Solid Edge part; units mm, degrees
sketch "Sketch1" plane through (0, 0, 0) normal (0, -1, 0) x (1, 0, 0)
  line L0 (-6.3509, -11) -> (6.3509, -11)
  line L1 (6.3509, -11) -> (12.7017, 0)
  line L2 (12.7017, 0) -> (6.3509, 11)
  line L3 (6.3509, 11) -> (-6.3509, 11)
  line L4 (-6.3509, 11) -> (-12.7017, 0)
  line L5 (-12.7017, 0) -> (-6.3509, -11)
extrude "Protrusion1" add sketch "Sketch1" along normal mid plane 16
sketch "Sketch2" plane through (0, 0, 0) normal (1, 0, 0) x (0, 1, 0)
  line L0 (8, -10) -> (7.2508, -12.391)
revolve "RevolvedCutout1" cut sketch "Sketch2" angle 360 about axis through (0, -63.5, 0) along (0, 1, 0) material side at (0, 7.6731, -11.2105)
mirror "Mirror1" about plane through (0, 0, 0) normal (0, -1, 0) of "RevolvedCutout1"
sketch "Sketch3" plane through (0, 0, 0) normal (1, 0, 0) x (0, 1, 0)
  line L0 (-8, -7.5) -> (-1.9048, -7.5)
  line L1 (-1.9048, -7.5) -> (-1.9048, -6)
  line L2 (-1.9048, -6) -> (7.1535, -6)
revolve "RevolvedCutout3" cut sketch "Sketch3" angle 360 about axis through (0, 7.1535, 0) along (0, -1, 0) material side at (0, -4.9524, -7.45)
Verification items for the finished model (mm, model axes). A direction names the side the tool comes from. Give positions to 0.01 mm unless a question says otherwise; leave off trailing zeros. Order: outer loops, then holes, each group sorted by start corner. A loop starts at its lowest first (then second) coordinate and runs counter-clockwise, first axis right, second up. Notation, with made-up numbers: M -21.75,65 L 22.25,65 A31 ccw 22.25,90 Z; hole C -18,0.5 d10. An arc over 180 degrees is marked long. Answer in a Markdown table with one row per item. Add a question column.
Item 1: Gauge pin test, flat ends, axial feed: pin 1 (7.5 mm diameter, centred on x = 3, z = 1, fed in from -Y); pin 2 (8 mm diameter, centred on x = 9, z = -7, fed in from -Y); pin 3 (4 mm diameter, centred on x = 8.5, y = -3, fed in from -Z). Record the tip position at first contact, or that the pin passes through.
Item 2: Scan lines: probe 1 along Z at (x, y) = (0, 5.25); probe 2 along Z at (x, y) = (-1.5, 5.5); probe 3 along X at (y, z) = (0.5, -1.75). Record each from-to range of solid material in increasing order. Write a range as from..to.
Item 3: Mould release check, pull along X, two halves, no side actions. Record for faces 3 (the flat face through (-9.571, 0.108, -5.423)), 4 (the cylindrical face through (-0.33, -4.91, 7.493)), 5 (the flat face through (0, 0, 11)): released by +X, released by -X, zero draft, split by the parting line, or undercut.
Item 4: Section check A-A, the plane x = 0. Enter the section's corners in (y, z).
Item 5: Section check B-B, the plane y = 3.25. Enter the section's corners in (x, z), and give its area (3 significant figures).
Item 6: Tool access check on faces 1 (the cylindrical face through (0, 3, 6)), 2 (the flat face through (6, -1.905, -2)). Record the directions out of +Z, -Z, +X, -X, +Y, -Y that give a thin tool (end or side, any length) a straight path to the whole face; none if there is none.
Filled sheet:
| question | item | result |
|---|---|---|
| 1 | pin 1 | stops at y = -1.9 |
| 1 | pin 2 | stops at y = -8 |
| 1 | pin 3 | stops at z = -10.74 |
| 2 | probe 1 | z = -11..-6, 6..11 |
| 2 | probe 2 | z = -11..-5.81, 5.81..11 |
| 2 | probe 3 | x = -11.69..-5.74, 5.74..11.69 |
| 3 | face 3 | released by -X |
| 3 | face 4 | undercut |
| 3 | face 5 | zero draft |
| 4 | outline | M -8,-10 L -7.69,-11 L 7.69,-11 L 8,-10 L 8,-6 L -1.9,-6 L -1.9,-7.5 L -8,-7.5 Z; M -8,7.5 L -1.9,7.5 L -1.9,6 L 8,6 L 8,10 L 7.69,11 L -7.69,11 L -8,10 Z |
| 5 | outline | M -12.7,0 L -6.35,-11 L 6.35,-11 L 12.7,0 L 6.35,11 L -6.35,11 Z; hole C 0,0 d12 |
| 5 | area | 306 mm^2 |
| 6 | face 1 | +Y, -Y |
| 6 | face 2 | -Y |
